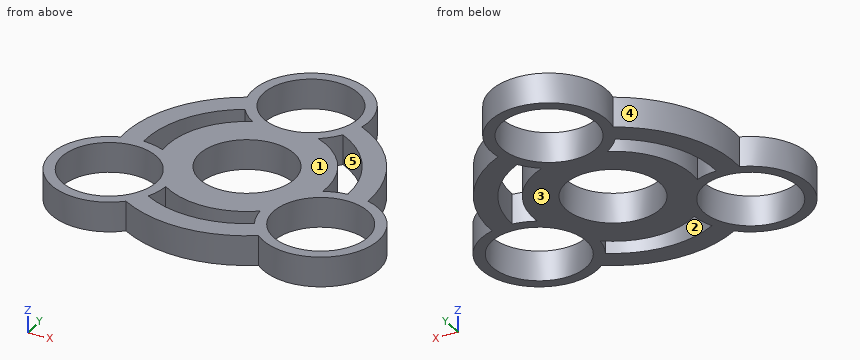
```python
from build123d import *

# Parameters (mm, degrees)
F0_R     = 11.05
F0_R_2   = 13.55
F1_DEPTH = 7


with BuildPart() as f1:
    # F0 (on Top) → F1 (new body)
    with BuildSketch(Plane.XY):
        with BuildLine():
            ThreePointArc((28.525726, -1.177043), (24.725025, 14.275), (13.243514, 25.292525))
            ThreePointArc((13.243514, 25.292525), (0, 41.708154), (-13.243514, 25.292525))
            ThreePointArc((-13.243514, 25.292525), (-24.725025, 14.275), (-28.525726, -1.177043))
            ThreePointArc((-28.525726, -1.177043), (-36.120321, -20.854077), (-15.282212, -24.115482))
            ThreePointArc((-15.282212, -24.115482), (0, -28.55), (15.282212, -24.115482))
            ThreePointArc((15.282212, -24.115482), (36.120321, -20.854077), (28.525726, -1.177043))
        make_face()
        with Locations((-24.385677, -14.079077)):
            Circle(F0_R, mode=Mode.SUBTRACT)
        with BuildLine():
            ThreePointArc((12.252611, -20.111589), (0, -23.55), (-12.252611, -20.111589))
            ThreePointArc((-12.252611, -20.111589), (-11.311855, -17.639648), (-10.869229, -15.032044))
            ThreePointArc((-10.869229, -15.032044), (0, -18.55), (10.869229, -15.032044))
            ThreePointArc((10.869229, -15.032044), (11.311855, -17.639648), (12.252611, -20.111589))
        make_face(mode=Mode.SUBTRACT)
        with Locations((24.385677, -14.079077)):
            Circle(F0_R, mode=Mode.SUBTRACT)
        Circle(F0_R_2, mode=Mode.SUBTRACT)
        with BuildLine():
            ThreePointArc((-23.543453, -0.555277), (-20.394898, 11.775), (-11.290842, 20.666867))
            ThreePointArc((-11.290842, 20.666867), (-9.620456, 18.616177), (-7.583517, 16.929051))
            ThreePointArc((-7.583517, 16.929051), (-16.064771, 9.275), (-18.452747, -1.897007))
            ThreePointArc((-18.452747, -1.897007), (-20.932311, -0.976529), (-23.543453, -0.555277))
        make_face(mode=Mode.SUBTRACT)
        with BuildLine():
            ThreePointArc((23.543453, -0.555277), (20.932311, -0.976529), (18.452747, -1.897007))
            ThreePointArc((18.452747, -1.897007), (16.064771, 9.275), (7.583517, 16.929051))
            ThreePointArc((7.583517, 16.929051), (9.620456, 18.616177), (11.290842, 20.666867))
            ThreePointArc((11.290842, 20.666867), (20.394898, 11.775), (23.543453, -0.555277))
        make_face(mode=Mode.SUBTRACT)
        with Locations((0, 28.158154)):
            Circle(F0_R, mode=Mode.SUBTRACT)
        Circle(F0_R_2)
        Circle(F0_R, mode=Mode.SUBTRACT)
    extrude(amount=F1_DEPTH)


solid = f1.part
```
Geometry: final body of the model. Coordinates: model frame, mm. Face numbers are marked on the shaded views. A direction names the side the tool comes from. Round coordinates to 2 decimals unless told otherwise and drop trailing zeros. Order: outer loops, then holes, each group sorted by start corner. A loop starts at its lowest first (then second) coordinate and runs counter-clockwise, first axis right, second up. Notation, with made-up numbers: (63, 15) -> (97, 15) arc R26 cw to (97, 35) -> close; hole circle Ø11 at (29.25, 4.5). An arc over 180 degrees is marked (long way). Write each question's results on one line, items separated by ' | '.
Q1. Pull-direction query (X, two-part tool) for the marked faces 3, 4 and 5; classes: released by +X, released by -X, zero draft, split by the parting line, or undercut.
Response values:
face 3: zero draft | face 4: released by -X | face 5: undercut
Q2. Access query for the marked faces 1 and 2. Directions: +Z, -Z, +X, -X, +Y, -Y. A direction counts if a zero-diameter tool reaches every point of the face in a straight line with its end or side. Return the directions, or none.
Response values:
face 1: +Z, +X, -X, +Y, -Y | face 2: +Z, -Z
Q3. Section query B-B (y = 7). Output: boundary loops of the cut face in (x, z).
Response values:
outline: (-27.68, 0) -> (-22.49, 0) -> (-22.49, 7) -> (-27.68, 7) -> close; (-17.18, 0) -> (-8.55, 0) -> (-8.55, 7) -> (-17.18, 7) -> close; (8.55, 0) -> (17.18, 0) -> (17.18, 7) -> (8.55, 7) -> close; (22.49, 0) -> (27.68, 0) -> (27.68, 7) -> (22.49, 7) -> close
Q4. Section query A-A (x = 0). Output: boundary loops of the cut face in (y, z).
Response values:
outline: (-28.55, 0) -> (-23.55, 0) -> (-23.55, 7) -> (-28.55, 7) -> close; (-18.55, 0) -> (-11.05, 0) -> (-11.05, 7) -> (-18.55, 7) -> close; (11.05, 0) -> (17.11, 0) -> (17.11, 7) -> (11.05, 7) -> close; (39.21, 0) -> (41.71, 0) -> (41.71, 7) -> (39.21, 7) -> close
Q5. Pin query (flat end, axial travel): pin 1 Ø5 at (x, y) = (4, 22.5) entering from +Z; pin 2 Ø12 at (x, y) = (5.5, 33.5) entering from -Z; pin 3 Ø1 at (x, z) = (-19.5, 1) entering from +Y; pin 4 Ø2 at (y, z) = (22, 2.5) entering from +X. Return the tip coordinate at first contact, or that it passes through.
Response values:
pin 1: through | pin 2: z = 0 | pin 3: y = 21.31 | pin 4: x = 19.34
Q6. Section query C-C (z = 2.25). Output: boundary loops of the cut face in (x, y), and give its area (3 significant figures).
Response values:
outline: (-28.53, -1.18) arc R13.55 ccw (long way) to (-15.28, -24.12) arc R28.55 ccw to (15.28, -24.12) arc R13.55 ccw (long way) to (28.53, -1.18) arc R28.55 ccw to (13.24, 25.29) arc R13.55 ccw (long way) to (-13.24, 25.29) arc R28.55 ccw to start; hole circle Ø22.1 at (-24.39, -14.08); hole (-23.54, -0.56) arc R13.55 cw to (-18.45, -1.9) arc R18.55 cw to (-7.58, 16.93) arc R13.55 cw to (-11.29, 20.67) arc R23.55 ccw to start; hole (-12.25, -20.11) arc R23.55 ccw to (12.25, -20.11) arc R13.55 cw to (10.87, -15.03) arc R18.55 cw to (-10.87, -15.03) arc R13.55 cw to start; hole circle Ø22.1 at (0, 0); hole circle Ø22.1 at (0, 28.16); hole (7.58, 16.93) arc R18.55 cw to (18.45, -1.9) arc R13.55 cw to (23.54, -0.56) arc R23.55 ccw to (11.29, 20.67) arc R13.55 cw to start; hole circle Ø22.1 at (24.39, -14.08) | area: 1,590 mm²
Q7. Section query D-D (y = -17). Output: boundary loops of the cut face in (x, z), and give its area (3 significant figures).
Response values:
outline: (-37.62, 0) -> (-35.04, 0) -> (-35.04, 7) -> (-37.62, 7) -> close; (-13.73, 0) -> (-11.15, 0) -> (-11.15, 7) -> (-13.73, 7) -> close; (-7.42, 0) -> (7.42, 0) -> (7.42, 7) -> (-7.42, 7) -> close; (11.15, 0) -> (13.73, 0) -> (13.73, 7) -> (11.15, 7) -> close; (35.04, 0) -> (37.62, 0) -> (37.62, 7) -> (35.04, 7) -> close | area: 176 mm²
Q8. Ray query, line 1 along Y through (x, z) = (0, 2); line 2 along Y through (x, z) = (-15, 6); line 3 along X through (y, z) = (-8.5, 4.25). Return the intervals inside material, ascending.
Response values:
line 1: -28.55 to -23.55, -18.55 to -11.05, 11.05 to 17.11, 39.21 to 41.71 | line 2: -24.29 to -19.91, -8.25 to 10.91, 18.15 to 24.29 | line 3: -36.73 to -33.92, -14.85 to -7.06, 7.06 to 14.85, 33.92 to 36.73
